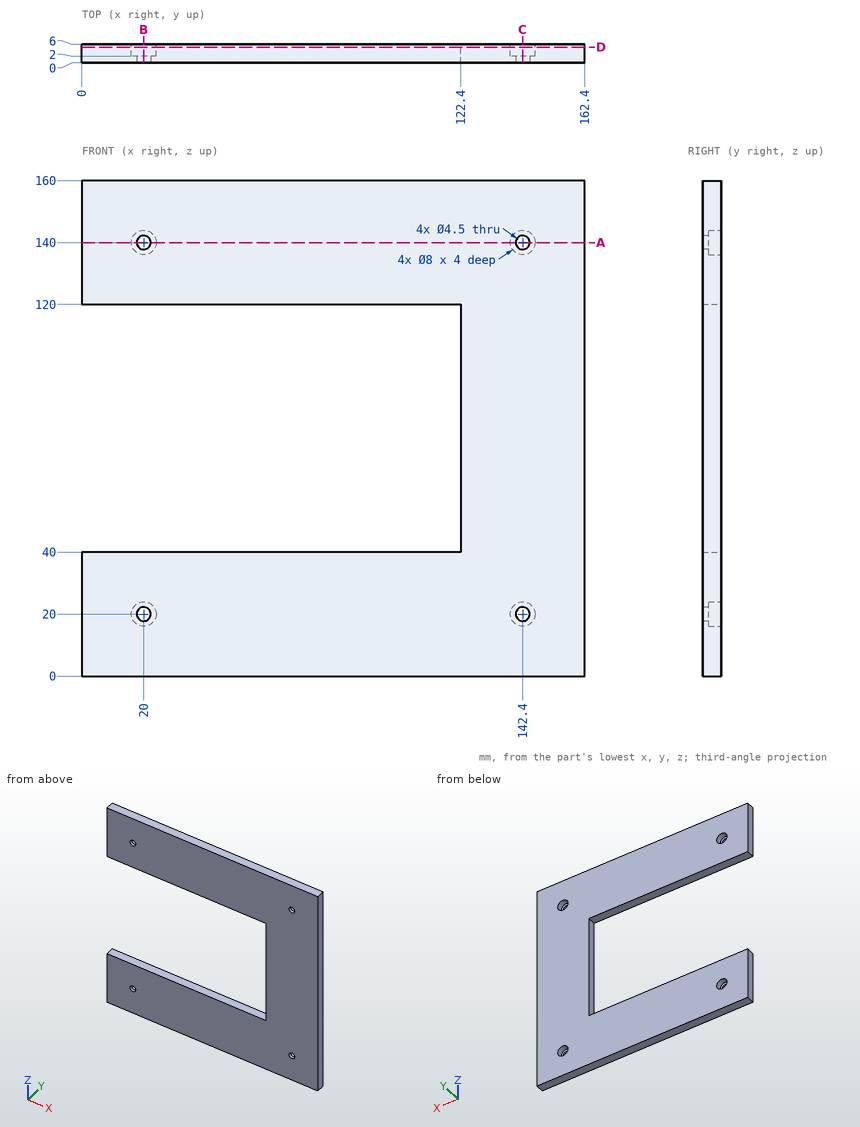
Print and shaded views of the part. All mm, measured from the part's lowest x, y and z. Coordinates: 2 decimals unless noted, no trailing zeros. Write each loop counter-clockwise with the first axis right and the second up, starting at its lowest first coordinate (ties: lowest second). Pieces come first, ordered by that corner, then holes. Notation, with made-up numbers: (65.5, 62) - (96.5, 62) arc R18 cw to (96.5, 73) - close; hole circle Ø5 at (80, 64). An arc over 180 degrees is marked (long way). One line per question, with ' | ' between items. Start each with the question number.
Q1. Cut at C-C, the plane x = 142.4. List the corners of the cut face in (y, z).
Q2. Cut at A-A, the plane z = 140. List the corners of the cut face in (x, y), then the cut area to 3 significant figures.
Q3. Cut at B-B, the plane x = 20. List the corners of the cut face in (y, z), then the cut area to 3 significant figures.
Q4. Pin check, flat tips, straight feed: pin 1 (4 mm diameter, centred on x = 20, z = 20, fed in from -Y); pin 2 (7 mm diameter, centred on x = 20, z = 20, fed in from +Y); pin 3 (3 mm diameter, centred on y = 4, z = 77, fed in from -X). Stop position of each tip, or through.
Q5. Cut at D-D, the plane y = 5. List the corners of the cut face in (x, z), then the cut area to 3 significant figures.
Q6. Drill centre lines: line 1 (Z direction, x = 142.4, y = 0.4); line 2 (X direction, y = 4, z = 20); line 3 (X direction, y = 1.65, z = 20). Where is each one in solid material? Low to high. Write a range as [from, to].
Answer below:
1) outline: (0, 0) - (6, 0) - (6, 16) - (2, 16) - (2, 17.75) - (0, 17.75) - close; (0, 22.25) - (2, 22.25) - (2, 24) - (6, 24) - (6, 136) - (2, 136) - (2, 137.75) - (0, 137.75) - close; (0, 142.25) - (2, 142.25) - (2, 144) - (6, 144) - (6, 160) - (0, 160) - close
2) outline: (0, 0) - (17.75, 0) - (17.75, 2) - (16, 2) - (16, 6) - (0, 6) - close; (22.25, 0) - (140.15, 0) - (140.15, 2) - (138.4, 2) - (138.4, 6) - (24, 6) - (24, 2) - (22.25, 2) - close; (144.65, 0) - (162.4, 0) - (162.4, 6) - (146.4, 6) - (146.4, 2) - (144.65, 2) - close | area: 892 mm^2
3) outline: (0, 0) - (6, 0) - (6, 16) - (2, 16) - (2, 17.75) - (0, 17.75) - close; (0, 22.25) - (2, 22.25) - (2, 24) - (6, 24) - (6, 40) - (0, 40) - close; (0, 120) - (6, 120) - (6, 136) - (2, 136) - (2, 137.75) - (0, 137.75) - close; (0, 142.25) - (2, 142.25) - (2, 144) - (6, 144) - (6, 160) - (0, 160) - close | area: 398 mm^2
4) pin 1: through | pin 2: y = 2 | pin 3: x = 122.4
5) outline: (0, 0) - (162.4, 0) - (162.4, 160) - (0, 160) - (0, 120) - (122.4, 120) - (122.4, 40) - (0, 40) - close; hole circle Ø8 at (20, 20); hole circle Ø8 at (20, 140); hole circle Ø8 at (142.4, 20); hole circle Ø8 at (142.4, 140) | area: 16,000 mm^2
6) line 1: [0, 17.75], [22.25, 137.75], [142.25, 160] | line 2: [0, 16], [24, 138.4], [146.4, 162.4] | line 3: [0, 17.75], [22.25, 140.15], [144.65, 162.4]
